CAD build for the part. Positions are in the model's coordinates, mm. A direction names the side the tool comes from. Give positions to 0.01 mm unless a question says otherwise; leave off trailing zeros. Order: outer loops, then holes, each group sorted by start corner. A loop starts at its lowest first (then second) coordinate and runs counter-clockwise, first axis right, second up. Notation, with made-up numbers: (52.5, 35.25) -> (86.5, 35.25) arc R21 ccw to (86.5, 71.25) -> close; hole circle Ø9 at (-3, 22). An arc over 180 degrees is marked (long way). Use one line per item in the form item = value. Start each with the question number.
1) Tool access for faces 4 (the face through (0, -23, 0)), 5 (the face through (0, 0, 0.794)), 6 (the face through (3.969, 22, -3)): list every direction of +Z, -Z, +X, -X, +Y, -Y with a clear straight run to the whole face (end or side of a thin tool).
2) Mould opens along Y. For faces 1 (the face through (-3.969, 22, -3)), 2 (the face through (0, 25.4, -1)), 3 (the face through (0, 19.05, -3)) say: pulls with the +Y half, pulls with the -Y half, needs draft (parallel to the pull), parting line crosses it, or undercut.
3) Cut at C-C, the plane y = 6. Give the cut face in (x, z).
4) Cut at B-B, the plane x = 7.5. Give the cut face in (y, z), and give its area (3 significant figures).
5) Cut at A-A, the plane z = -5. Give the cut face in (x, y), and give its area (3 significant figures).
6) Drop flat-ended pins along their axis: P1, Ø4.5, axis at y = 22.22, z = -5.56, coming from the -X side; P2, Ø1.9, axis at x = -1, z = -3, coming from the -Y side; P3, Ø1.9, axis at y = 23, z = -4.5, coming from the +X side. Give the stop position or say it passes through.
7) Probe line 1 (Y direction, x = -3.5, z = -5.75); line 2 (Z direction, x = 26.5, y = 16); line 3 (Y direction, x = 1, z = -4). List the from-to ranges inside material, lowest first.
from build123d import *

# Parameters (mm, degrees)
SKETCH1_W                = 66.675
SKETCH1_H                = 50.8
BOSS_EXTRUDE1_DEPTH      = 0.79375
BOSS_EXTRUDE2_DEPTH      = 3.96875
M3_CLEARANCE_HOLE2_D     = 3.4
M3_CLEARANCE_HOLE2_DEPTH = 6.35
M3_CLEARANCE_HOLE2_TIP   = 1.021463052
SKETCH11_W               = 66.675
SKETCH11_H               = 6.35
BOSS_EXTRUDE3_DEPTH      = 1.5875


with BuildPart() as part:
    # Sketch1 → Boss-Extrude1 (new body)
    with BuildSketch(Plane.XY):
        Rectangle(SKETCH1_W, SKETCH1_H)
    extrude(amount=BOSS_EXTRUDE1_DEPTH)

    # Sketch3 → Boss-Extrude2 (add, symmetric)
    with BuildSketch(Plane(origin=(0, 0, 0), x_dir=(0, 0, -1), z_dir=(1, 0, 0))):
        with BuildLine():
            Line((0, 25.4), (6.19125, 25.4))
            ThreePointArc((6.19125, 25.4), (7.987301224, 24.656051224), (8.73125, 22.86))
            Line((8.73125, 22.86), (8.73125, 21.59))
            ThreePointArc((8.73125, 21.59), (7.987301224, 19.793948776), (6.19125, 19.05))
            Line((6.19125, 19.05), (0, 19.05))
            Line((0, 19.05), (0, 25.4))
        make_face()
    extrude(amount=BOSS_EXTRUDE2_DEPTH, both=True)

    # Sketch8 → M3 Clearance Hole1 (revolve, cut)
    with BuildSketch(Plane(origin=(0, 22.225, -5.55625), x_dir=(0, 0, -1), z_dir=(0, 1, 0))):
        Polygon((0, 0), (0, 7.371463052), (1.7, 6.35), (1.7, 0), align=None)
    revolve(axis=Axis((6.35, 22.225, -5.55625), (-1, 0, 0)), mode=Mode.SUBTRACT)

    # M3 Clearance Hole2
    with Locations(Plane.ZY):
        with Locations((-5.55625, 22.225)):
            Hole(M3_CLEARANCE_HOLE2_D / 2, depth=M3_CLEARANCE_HOLE2_DEPTH)
            with Locations((0, 0, -(M3_CLEARANCE_HOLE2_DEPTH + M3_CLEARANCE_HOLE2_TIP / 2))):  # 118° drill point
                Cone(0, M3_CLEARANCE_HOLE2_D / 2, M3_CLEARANCE_HOLE2_TIP, mode=Mode.SUBTRACT)

    # Sketch11 → Boss-Extrude3 (add)
    with BuildSketch(Plane(origin=(0, 0, 0), x_dir=(-1, 0, 0), z_dir=(0, 0, -1))):
        with Locations((0, -17.4625)):
            Rectangle(SKETCH11_W, SKETCH11_H)
    extrude(amount=BOSS_EXTRUDE3_DEPTH)


solid = part.part
Result:
q1.face_4 = -Z, +X, -X, -Y
q1.face_5 = +Z, +X, -X, +Y, -Y
q1.face_6 = -Z, +X, +Y
q2.face_1 = needs draft
q2.face_2 = pulls with the +Y half
q2.face_3 = undercut
q3.outline = (-33.34, 0) -> (33.34, 0) -> (33.34, 0.79) -> (-33.34, 0.79) -> close
q4.outline = (-25.4, 0) -> (-20.64, 0) -> (-20.64, -1.59) -> (-14.29, -1.59) -> (-14.29, 0) -> (25.4, 0) -> (25.4, 0.79) -> (-25.4, 0.79) -> close
q4.area = 50.4 mm²
q5.outline = (-3.97, 19.05) -> (3.97, 19.05) -> (3.97, 20.62) -> (-3.97, 20.62) -> close; (-3.97, 23.83) -> (3.97, 23.83) -> (3.97, 25.4) -> (-3.97, 25.4) -> close
q5.area = 24.9 mm²
q6.P1 = -3.97
q6.P2 = 19.05
q6.P3 = 3.97
q7.line_1 = 19.05 to 20.54, 23.91 to 25.4
q7.line_2 = 0 to 0.79
q7.line_3 = 19.05 to 21.54, 22.91 to 25.4
